from build123d import *

# Parameters (mm, degrees)
F1_DEPTH = 12.7
F3_DEPTH = 1.5875
F4_R     = 1.7145
F5_DEPTH = 25.4


with BuildPart() as f1:
    # F0 (on Front) → F1 (new body, symmetric)
    with BuildSketch(Plane.XZ):
        with BuildLine():
            ThreePointArc((-12.6841150657, 0.635), (0, 12.7), (12.6841150657, 0.635))
            Line((12.6841150657, 0.635), (22.2091150657, 0.635))
            Line((22.2091150657, 0.635), (22.2091150657, 3.175))
            Line((22.2091150657, 3.175), (15.5542598667, 3.175))
            ThreePointArc((15.5542598667, 3.175), (0, 15.875), (-15.5542598667, 3.175))
            Line((-15.5542598667, 3.175), (-22.2091150657, 3.175))
            Line((-22.2091150657, 3.175), (-22.2091150657, 0.635))
            Line((-22.2091150657, 0.635), (-22.2091150657, 0))
            Line((-22.2091150657, 0), (-12.7, 0))
            ThreePointArc((-12.7, 0), (-12.6960281453, 0.3175993274), (-12.6841150657, 0.635))
        make_face()
    extrude(amount=F1_DEPTH, both=True)

    # F2 (on Front) → F3 (join, symmetric)
    with BuildSketch(Plane.XZ):
        with BuildLine():
            ThreePointArc((-15.5542598667, 3.175), (-14.6349663523, 6.1508848848), (-13.1523201375, 8.89))
            Line((-13.1523201375, 8.89), (-50.8, 8.89))
            ThreePointArc((-50.8, 8.89), (-55.2901280605, 7.0301280605), (-57.15, 2.54))
            Line((-57.15, 2.54), (-57.15, 0))
            Line((-57.15, 0), (-53.975, 0))
            ThreePointArc((-53.975, 0), (-50.8, 3.175), (-47.625, 0))
            Line((-47.625, 0), (-22.2091150657, 0))
            Line((-22.2091150657, 0), (-22.2091150657, 3.175))
            Line((-22.2091150657, 3.175), (-15.5542598667, 3.175))
        make_face()
    extrude(amount=F3_DEPTH, both=True)

    # F4 (on face) → F5 (cut)
    with BuildSketch(Plane.XY.offset(3.175)):
        with Locations((19.1611150657, 8.89)):
            Circle(F4_R)
        with Locations((19.1611150657, -8.89)):
            Circle(F4_R)
        with Locations((-19.1611150657, -8.89)):
            Circle(F4_R)
        with Locations((-19.1611150657, 8.89)):
            Circle(F4_R)
    extrude(amount=-F5_DEPTH, mode=Mode.SUBTRACT)


solid = f1.part
Could you check a few things on this model? Use its own coordinates, in mm. A direction names the side the tool comes from. Coordinates: 2 decimals unless noted, no trailing zeros. Loops run counter-clockwise (first coordinate to the right, second up) from the corner with the lowest first, then second, coordinate; pieces in that order, holes last.
1. For faces 5 (the face through (-22.209, -7, 2)), 6 (the face through (17, 0, 0.635)), 7 (the face through (-19, 7, 3.175)), 8 (the face through (-22.209, 7, 2)), 9 (the face through (-18, -7, 3.175)), which set-ups out of +Z, -Z, +X, -X, +Y, -Y let a thin tool reach every point of the face, with its end or its side?
2. Imagine slicing it at A-A (y = -8.89). Please give me the cut outline in (x, z) (3 decimals).
3. I need wall thicknesses on L1, parallel to X at y = -9.75, z = 2.5; L2, parallel to Y at x = -16.5, z = 5; L3, parallel to Z at x = -27, y = 1.25. Which ranges of each line are inside material? Lowest first, please.
4. For P1, Ø2, axis at x = -20.5, y = 5.5, coming from the +Z side (3 decimals); P2, Ø4.5, axis at x = 19.16, y = 8.89, coming from the -Z side (3 decimals); P3, Ø1.6, axis at y = 9, z = 1.5, coming from the -X side; P4, Ø4.5, axis at x = -19.16, y = 8.89, coming from the -Z side, each with a flat end and sliding along its axis, tell me the tip position at first contact or that it passes through.
5. Imagine slicing it at C-C (z = 11). Please give me the cut outline in (x, y), and give its area (3 significant figures).
6. Imagine slicing it at B-B (z = 1.75). Please give me the cut outline in (x, y).
7. We'd pull the mould along Y, two halves only. Please class faces 1 (the face through (22.209, 0, 2)), 2 (the face through (0, 12.7, 13)), 3 (the face through (-20.425, 10.049, 1.61)), 4 (the face through (0, -12.7, 13)): released by +Y, released by -Y, zero draft, split by the parting line, or undercut.
8. Imagine slicing it at D-D (y = 0). Please give me the cut outline in (x, z) (3 decimals), and give its area (3 significant figures).
Computed values:
1. face 5: +Z, -Z, -X, -Y
1. face 6: -Z, +X, +Y, -Y
1. face 7: +Z, -X, +Y
1. face 8: +Z, -Z, -X, +Y
1. face 9: +Z, -X, -Y
2. outline: (-22.209, 0) - (-20.876, 0) - (-20.876, 3.175) - (-22.209, 3.175) - close; (-17.447, 0) - (-12.7, 0) arc R12.7 cw to (12.684, 0.635) - (17.447, 0.635) - (17.447, 3.175) - (15.554, 3.175) arc R15.875 ccw to (-15.554, 3.175) - (-17.447, 3.175) - close; (20.876, 0.635) - (22.209, 0.635) - (22.209, 3.175) - (20.876, 3.175) - close
3. L1: x = -22.21 to -20.64, -17.68 to -12.45, 12.45 to 17.68, 20.64 to 22.21
3. L2: y = -1.59 to 1.59
3. L3: z = 0 to 8.89
4. P1: stops at z = 3.175
4. P2: stops at z = 0.635
4. P3: stops at x = -22.21
4. P4: stops at z = 0
5. outline: (-11.45, -12.7) - (-6.35, -12.7) - (-6.35, 12.7) - (-11.45, 12.7) - close; (6.35, -12.7) - (11.45, -12.7) - (11.45, 12.7) - (6.35, 12.7) - close
5. area: 259 mm2
6. outline: (-57.15, -1.59) - (-53.45, -1.59) - (-53.45, 1.59) - (-57.15, 1.59) - close; (-48.15, -1.59) - (-22.21, -1.59) - (-22.21, -12.7) - (-12.58, -12.7) - (-12.58, 12.7) - (-22.21, 12.7) - (-22.21, 1.59) - (-48.15, 1.59) - close; (12.58, -12.7) - (22.21, -12.7) - (22.21, 12.7) - (12.58, 12.7) - close; hole circle Ø3.43 at (-19.16, -8.89); hole circle Ø3.43 at (-19.16, 8.89); hole circle Ø3.43 at (19.16, -8.89); hole circle Ø3.43 at (19.16, 8.89)
7. face 1: zero draft
7. face 2: released by +Y
7. face 3: undercut
7. face 4: released by -Y
8. outline: (-57.15, 0) - (-53.975, 0) arc R3.175 cw to (-47.625, 0) - (-12.7, 0) arc R12.7 cw to (12.684, 0.635) - (22.209, 0.635) - (22.209, 3.175) - (15.554, 3.175) arc R15.875 ccw to (-13.152, 8.89) - (-50.8, 8.89) arc R6.35 ccw to (-57.15, 2.54) - close
8. area: 507 mm2
